Source: CAD feature listing. Evaluate the final solid. Frame: model axes, mm. A direction names the side the tool comes from. Give positions to 0.01 mm unless a question says otherwise; leave off trailing zeros. Order: outer loops, then holes, each group sorted by start corner. A loop starts at its lowest first (then second) coordinate and runs counter-clockwise, first axis right, second up. Notation, with made-up numbers: M -10,3 L 10,3 A26 ccw 10,27 Z; hole C -28.5,29 d6. An arc over 180 degrees is marked long. Answer in a Markdown table with one row per item. Add a question column.
(1) Section query B-B, the plane z = 125. Return loops of the section in (x, y), plus the area to 3 significant figures.
(2) Set-up query: faces 1 (the face through (-1, -141.288, 86)), 2 (the face through (-66.675, -2, 5)). Return all of +Z, -Z, +X, -X, +Y, -Y with unobstructed straight access to the full face (end or side cutting, diameter ignored); none if empty.
(3) Pin query (flat end, axial travel): P1, Ø8, axis at x = -40, y = 64, coming from the -Z side; P2, Ø12, axis at x = -23.5, y = -42, coming from the +Z side. Return the tip coordinate at first contact, or that it passes through.
(4) Material intervals for line 1 along Y through (x, z) = (-58.5, 159); line 2 along X through (y, z) = (101.5, 111.5); line 3 along Z through (x, y) = (-9, 11.5), sorted ascending.
(5) Section query A-A, the plane x = 0. Return loops of the section in (y, z) (1 decimal).
from build123d import *

# Parameters (mm, degrees)
F0_W     = 142.875
F0_H     = 282.575
F1_DEPTH = 174.625
F2_T     = -1.5875
F3_W     = 133.35
F3_H     = 273.05
F4_DEPTH = 6.35


with BuildPart() as f1:
    # F0 (on Top) → F1 (new body)
    with BuildSketch(Plane.XY):
        Rectangle(F0_W, F0_H)
    extrude(amount=F1_DEPTH)

    # F2
    f2_openings = [f1.faces().sort_by_distance(p)[0] for p in [
        (0, 0, 174.625),
    ]]
    offset(amount=F2_T, openings=f2_openings)

    # F3 (on face) → F4 (join)
    with BuildSketch(Plane.XY.offset(1.5875)):
        Rectangle(F3_W, F3_H)
    extrude(amount=F4_DEPTH)


solid = f1.part
Values follow:
| question | item | result |
|---|---|---|
| 1 | outline | M -71.44,-141.29 L 71.44,-141.29 L 71.44,141.29 L -71.44,141.29 Z; hole M -69.85,-139.7 L 69.85,-139.7 L 69.85,139.7 L -69.85,139.7 Z |
| 1 | area | 1,340 mm² |
| 2 | face 1 | +Z, -Z, +X, -X, -Y |
| 2 | face 2 | +Z |
| 3 | P1 | stops at z = 0 |
| 3 | P2 | stops at z = 7.94 |
| 4 | line 1 | y = -141.29 to -139.7, 139.7 to 141.29 |
| 4 | line 2 | x = -71.44 to -69.85, 69.85 to 71.44 |
| 4 | line 3 | z = 0 to 7.94 |
| 5 | outline | M -141.3,0 L 141.3,0 L 141.3,174.6 L 139.7,174.6 L 139.7,1.6 L 136.5,1.6 L 136.5,7.9 L -136.5,7.9 L -136.5,1.6 L -139.7,1.6 L -139.7,174.6 L -141.3,174.6 Z |
